Geometry: see drawing. Coordinates: mm, zero at the bounding-box minimum. A direction names the side the tool comes from. Coordinates: 2 decimals unless noted, no trailing zeros. Order: outer loops, then holes, each group sorted by start corner. A loop starts at its lowest first (then second) coordinate and runs counter-clockwise, first axis right, second up.
Item 1: Mould query, pull axis Z, two halves, no side actions, for the marked faces 1, 2 and 3. Classes: released by +Z, released by -Z, zero draft, split by the parting line, or undercut.
Item 2: Section D-D on x = 164.5. Return the cut outline in (y, z), then the cut area to 4 significant figures.
Item 3: Section B-B on x = 81.5. Return the cut outline in (y, z).
Item 4: Section A-A on z = 73. Return the cut outline in (x, y), then the cut area to 3 significant figures.
Item 5: Ray query, line 1 (Z direction, x = 76, y = 79); line 2 (Y direction, x = 164.5, z = 69); line 3 (X direction, y = 224, z = 54.5). Return the intervals inside material, ascending.
Item 6: Contact query for flat-ended pins moving along their axis: P1, Ø16.5, axis at x = 83.5, y = 198.5, coming from the +Z side; P2, Ø16.5, axis at x = 77, y = 125.5, coming from the -Z side; P3, Ø4, axis at y = 233.5, z = 56, coming from the +X side. Output: stop coordinate, or through.
Item 7: Section C-C on y = 41. Return the cut outline in (x, z), then the cut area to 3 significant figures.
Item 8: Reachability of the marked faces 4, 5, 6 and 7 from +Z, -Z, +X, -X, +Y, -Y: full face, straight path, thin tool, end or side. Return the list, or none.
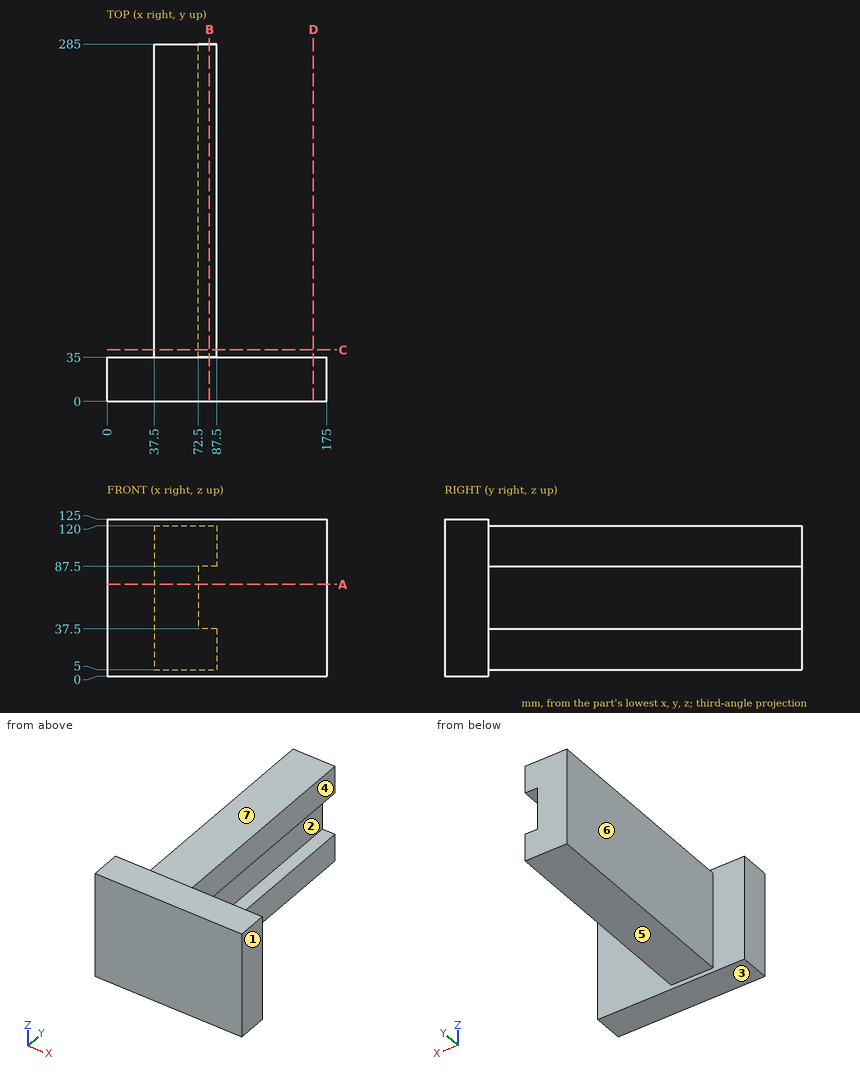
Answer list:
1. face 1: zero draft
1. face 2: undercut
1. face 3: released by -Z
2. outline: (0, 0) - (35, 0) - (35, 125) - (0, 125) - close
2. area: 4,375 mm2
3. outline: (0, 0) - (35, 0) - (35, 5) - (285, 5) - (285, 37.5) - (35, 37.5) - (35, 87.5) - (285, 87.5) - (285, 120) - (35, 120) - (35, 125) - (0, 125) - close
4. outline: (0, 0) - (175, 0) - (175, 35) - (72.5, 35) - (72.5, 285) - (37.5, 285) - (37.5, 35) - (0, 35) - close
4. area: 14,900 mm2
5. line 1: z = 5 to 37.5, 87.5 to 120
5. line 2: y = 0 to 35
5. line 3: x = 37.5 to 72.5
6. P1: stops at z = 120
6. P2: stops at z = 5
6. P3: stops at x = 72.5
7. outline: (37.5, 5) - (87.5, 5) - (87.5, 37.5) - (72.5, 37.5) - (72.5, 87.5) - (87.5, 87.5) - (87.5, 120) - (37.5, 120) - close
7. area: 5,000 mm2
8. face 4: +Z, -Z, +X, +Y
8. face 5: -Z, +X, -X, +Y
8. face 6: +Z, -Z, -X, +Y
8. face 7: +Z, +X, -X, +Y
